Input: part model. Units: mm. Frame: model coordinates. A direction names the side the tool comes from. Round coordinates to 2 decimals unless told otherwise and drop trailing zeros. Loops run counter-clockwise (first coordinate to the right, second up) from the corner with the lowest first, then second, coordinate; pieces in that order, holes last.
1) Section B-B, the plane y = -1.5. Return loops of the section in (x, z).
2) First-contact query: pin 1 (1.5 mm diameter, centred on x = 1, y = 1.5, fed in from -Z). Flat tip, straight axial feed; report the tip coordinate or a pass-through.
3) Section D-D, the plane z = 0.5. Return loops of the section in (x, y), and give its area (3 significant figures).
4) Access query for faces 1 (the face through (0, 0, 3.2)), 2 (the face through (-0.99, 1.75, 3.55)). Directions: +Z, -Z, +X, -X, +Y, -Y. A direction counts if a zero-diameter tool reaches every point of the face in a straight line with its end or side. Return the directions, or none.
5) Draft query along X for faces 3 (the face through (0.65, -0.27, 6.75)), 4 (the face through (1, 0, 10.2)), 5 (the face through (1.92, 0.6, 8.72)), 6 (the face through (1.02, 1.73, 3.55)). Return one class per face: pulls with the +X half, pulls with the -X half, needs draft (parallel to the pull), parting line crosses it, or undercut.
6) Section A-A, the plane z = 5.75. Return loops of the section in (x, y) (3 decimals), and give its area (3 significant figures).
7) Ray query, line 1 along Y through (x, z) = (0, 8) (3 decimals); line 2 along Z through (x, y) = (-0.15, -0.65); line 3 along Z through (x, y) = (1.75, 1.2). Return the intervals inside material, ascending.
from build123d import *

# Parameters (mm, degrees)
BOSS_EXTRUDE1_DEPTH = 10.2
SKETCH2_R           = 2.320948082
SKETCH2_R_2         = 2.01
CUT_EXTRUDE2_DEPTH  = 3
SKETCH4_R           = 0.705
CUT_EXTRUDE3_DEPTH  = 7


with BuildPart() as part:
    # Sketch1 → Boss-Extrude1 (new body)
    with BuildSketch(Plane.XY):
        Polygon((0, -2.320948082), (2.01, -1.160474041), (2.01, 1.160474041), (0, 2.320948082), (-2.01, 1.160474041), (-2.01, -1.160474041), align=None)
    extrude(amount=BOSS_EXTRUDE1_DEPTH)

    # Sketch2 → Cut-Extrude2 (cut)
    with BuildSketch(Plane.XY.offset(10.2)):
        Circle(SKETCH2_R)
        Circle(SKETCH2_R_2, mode=Mode.SUBTRACT)
    extrude(amount=-CUT_EXTRUDE2_DEPTH, mode=Mode.SUBTRACT)

    # Sketch4 → Cut-Extrude3 (cut)
    with BuildSketch(Plane.XY.offset(10.2)):
        Circle(SKETCH4_R)
    extrude(amount=-CUT_EXTRUDE3_DEPTH, mode=Mode.SUBTRACT)


solid = part.part
Final values:
1. outline: (-1.42, 0) - (1.42, 0) - (1.42, 7.2) - (1.34, 7.2) - (1.34, 10.2) - (-1.34, 10.2) - (-1.34, 7.2) - (-1.42, 7.2) - close
2. pin 1: stops at z = 0
3. outline: (-2.01, -1.16) - (0, -2.32) - (2.01, -1.16) - (2.01, 1.16) - (0, 2.32) - (-2.01, 1.16) - close
3. area: 14.0 mm2
4. face 1: +Z
4. face 2: +Z, -Z, -X, +Y
5. face 3: undercut
5. face 4: needs draft
5. face 5: parting line crosses it
5. face 6: pulls with the +X half
6. outline: (-2.01, -1.16) - (0, -2.321) - (2.01, -1.16) - (2.01, 1.16) - (0, 2.321) - (-2.01, 1.16) - close; hole circle Ø1.41 at (0, 0)
6. area: 12.4 mm2
7. line 1: y = -2.01 to -0.705, 0.705 to 2.01
7. line 2: z = 0 to 3.2
7. line 3: z = 0 to 7.2
